Input: dimensioned drawing with shaded views. Units: mm. Origin: part minimum x, y, z. Give positions to 0.01 mm unless a question says otherwise; leave off trailing zeros. Loops run counter-clockwise (first coordinate to the right, second up) from the corner with the lowest first, then second, coordinate; pieces in that order, holes last. Notation, with made-up numbers: (-26.75, 24) -> (-19.75, 24) arc R29 ccw to (-19.75, 53) -> close; hole circle Ø4 at (54.5, -26.75). An arc over 180 degrees is marked (long way). Answer in a Markdown table with one row per item. Add a question column.
1) Section query C-C (z = 1.5). Return the cut outline in (x, y), plus the area to 3 significant figures.
2) Section query D-D (y = 31.5). Return the cut outline in (x, z), plus the area to 3 significant figures.
3) Section query A-A (x = 23.75). Return the cut outline in (y, z).
4) Line query: line 1 (X direction, y = 23.75, z = 0.95); line 2 (X direction, y = 23.75, z = 1.35). Output: solid intervals per line, ascending. Write a range as from..to.
5) Draft query along Y for the marked faces 1 and 2. Return one class per face: +Y half, -Y half, draft (parallel to the pull), parting line (faces both ways), or undercut.
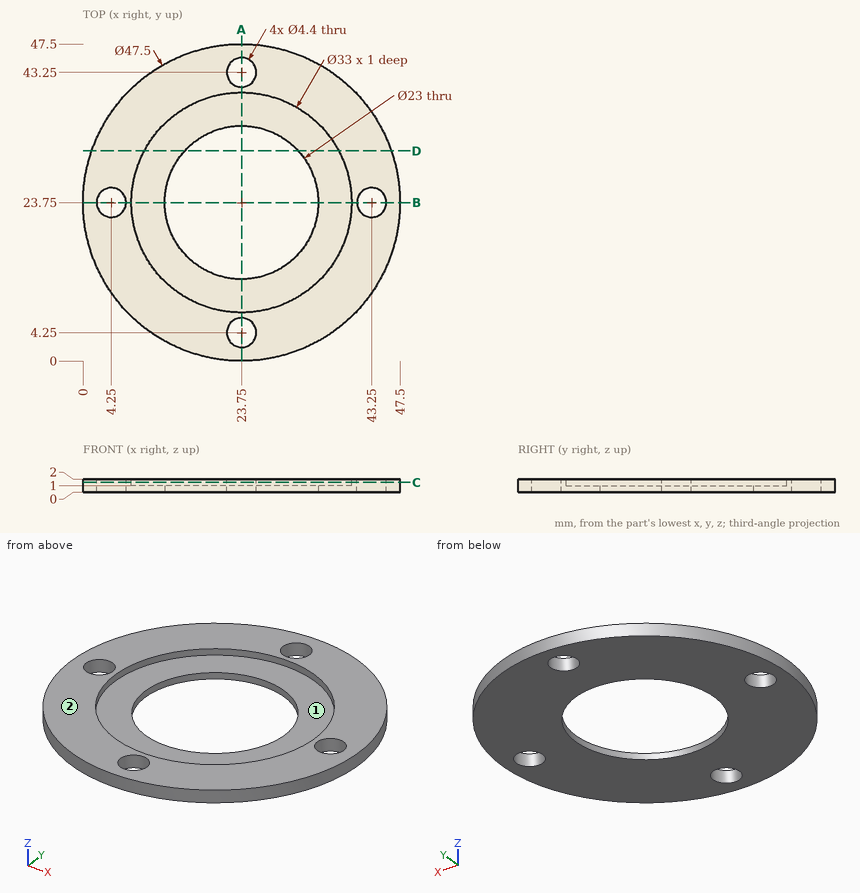
Evaluation:
| question | item | result |
|---|---|---|
| 1 | outline | circle Ø47.5 at (23.75, 23.75); hole circle Ø4.4 at (4.25, 23.75); hole circle Ø33 at (23.75, 23.75); hole circle Ø4.4 at (23.75, 4.25); hole circle Ø4.4 at (23.75, 43.25); hole circle Ø4.4 at (43.25, 23.75) |
| 1 | area | 856 mm² |
| 2 | outline | (1.3, 0) -> (15.25, 0) -> (15.25, 1) -> (9.18, 1) -> (9.18, 2) -> (1.3, 2) -> close; (32.25, 0) -> (46.2, 0) -> (46.2, 2) -> (38.32, 2) -> (38.32, 1) -> (32.25, 1) -> close |
| 2 | area | 43.7 mm² |
| 3 | outline | (0, 0) -> (2.05, 0) -> (2.05, 2) -> (0, 2) -> close; (6.45, 0) -> (12.25, 0) -> (12.25, 1) -> (7.25, 1) -> (7.25, 2) -> (6.45, 2) -> close; (35.25, 0) -> (41.05, 0) -> (41.05, 2) -> (40.25, 2) -> (40.25, 1) -> (35.25, 1) -> close; (45.45, 0) -> (47.5, 0) -> (47.5, 2) -> (45.45, 2) -> close |
| 4 | line 1 | 0..2.05, 6.45..12.25, 35.25..41.05, 45.45..47.5 |
| 4 | line 2 | 0..2.05, 6.45..7.25, 40.25..41.05, 45.45..47.5 |
| 5 | face 1 | undercut |
| 5 | face 2 | draft |
